Input: part model. Units: mm. Frame: model coordinates. A direction names the side the tool comes from. Coordinates: 2 decimals unless noted, no trailing zeros. Loops run counter-clockwise (first coordinate to the right, second up) from the corner with the lowest first, then second, coordinate; pieces in that order, holes last.
```python
from build123d import *

# Parameters (mm, degrees)
F0_R     = 5.3
F1_DEPTH = 3
F2_W     = 10.177304
F2_H     = 3
F3_DEPTH = 5
F4_R     = 1.5
F5_DEPTH = 5


with BuildPart() as f1:
    # F0 (on Top) → F1 (new body)
    with BuildSketch(Plane.XY):
        with BuildLine():
            Line((-12.261554, 0), (-20, 0))
            Line((-20, 0), (-20, -3))
            Line((-20, -3), (0, -3))
            Line((0, -3), (20, -3))
            Line((20, -3), (20, 0))
            Line((20, 0), (12.261554, 0))
            ThreePointArc((12.261554, 0), (8.853776, 1.888736), (7.485685, 5.536832))
            ThreePointArc((7.485685, 5.536832), (7.488618, 5.754393), (7.499947, 5.971679))
            ThreePointArc((7.499947, 5.971679), (0, 13.5), (-7.499947, 5.971679))
            ThreePointArc((-7.499947, 5.971679), (-7.488618, 5.754393), (-7.485685, 5.536832))
            ThreePointArc((-7.485685, 5.536832), (-8.853776, 1.888736), (-12.261554, 0))
        make_face()
        with Locations((0, 6)):
            Circle(F0_R, mode=Mode.SUBTRACT)
        with BuildLine():
            ThreePointArc((-7.499947, 5.971679), (-7.495969, 5.754152), (-7.485685, 5.536832))
            ThreePointArc((-7.485685, 5.536832), (-7.488618, 5.754393), (-7.499947, 5.971679))
        make_face()
        with BuildLine():
            ThreePointArc((7.485685, 5.536832), (7.495969, 5.754152), (7.499947, 5.971679))
            ThreePointArc((7.499947, 5.971679), (7.488618, 5.754393), (7.485685, 5.536832))
        make_face()
    extrude(amount=F1_DEPTH)

    # F2 (on face) → F3 (join)
    with BuildSketch(Plane(origin=(0, 0, 0), x_dir=(1, 0, 0), z_dir=(0, 0, -1))):
        with Locations((-14.911348, 1.5)):
            Rectangle(F2_W, F2_H)
        with Locations((14.911348, 1.5)):
            Rectangle(F2_W, F2_H)
    extrude(amount=F3_DEPTH)

    # F4 (on face) → F5 (cut)
    with BuildSketch(Plane(origin=(0, 0, 0), x_dir=(-1, 0, 0), z_dir=(0, 1, 0))):
        with Locations((-15, -2)):
            Circle(F4_R)
        with Locations((15, -2)):
            Circle(F4_R)
    extrude(amount=-F5_DEPTH, mode=Mode.SUBTRACT)


solid = f1.part
```
Item 1: Line query: L1, parallel to Z at x = 15, y = -1.75; L2, parallel to Y at x = 15.5, z = 0; L3, parallel to Y at x = 0, z = 1.55. Output: solid intervals per line, ascending.
Result:
L1: z = -5 to -3.5, -0.5 to 3
L2: y = -3 to 0
L3: y = -3 to 0.7, 11.3 to 13.5
Item 2: Section query D-D (y = 7.75). Output: boundary loops of the cut face in (x, z).
Result:
outline: (-7.29, 0) - (-5, 0) - (-5, 3) - (-7.29, 3) - close; (5, 0) - (7.29, 0) - (7.29, 3) - (5, 3) - close
Item 3: Reachability of faces 1 (the face through (-9.823, -1, -2)), 2 (the face through (-15, 0, 0)), 3 (the face through (16.5, -1.48, -1.93)) from +Z, -Z, +X, -X, +Y, -Y: full face, straight path, thin tool, end or side. Return the list, or none.
Result:
face 1: -Z, +Y, -Y
face 2: -Z, -X, +Y
face 3: +Y, -Y
Item 4: Contact query for flat-ended pins moving along their axis: P1, Ø2.5, axis at x = -13, z = -0.5, coming from the +Y side; P2, Ø1, axis at y = 1, z = 1, coming from the +X side; P3, Ø2, axis at x = -15, z = 1.5, coming from the +Y side; P4, Ø8, axis at x = 7.5, y = 1.5, coming from the -Z side. Output: stop coordinate, or through.
Result:
P1: stops at y = 0.08
P2: stops at x = 10.66
P3: stops at y = 0
P4: stops at z = -5
Item 5: Section query A-A (x = 15). Output: boundary loops of the cut face in (y, z), then the cut area to 3 significant figures.
Result:
outline: (-3, -5) - (0, -5) - (0, -3.5) - (-3, -3.5) - close; (-3, -0.5) - (0, -0.5) - (0, 3) - (-3, 3) - close
area: 15.0 mm2
Item 6: Mould query, pull axis Y, two halves, no side actions, for faces 4 (the face through (-13.5, -1.48, -1.93)), 5 (the face through (0, -3, 1)), 6 (the face through (-0.69, 11.255, 1.479)), 7 (the face through (15, 0, 0)). Classes: +Y half, -Y half, draft (parallel to the pull), parting line (faces both ways), or undercut.
Result:
face 4: draft
face 5: -Y half
face 6: undercut
face 7: +Y half
Item 7: Section query B-B (y = -1.75). Output: boundary loops of the cut face in (x, z).
Result:
outline: (-20, -5) - (-9.82, -5) - (-9.82, 0) - (9.82, 0) - (9.82, -5) - (20, -5) - (20, 3) - (-20, 3) - close; hole circle Ø3 at (-15, -2); hole circle Ø3 at (15, -2)
Item 8: Section query C-C (z = -1). Output: boundary loops of the cut face in (x, y), then the cut area to 3 significant figures.
Result:
outline: (-20, -3) - (-16.12, -3) - (-16.12, 0) - (-20, 0) - close; (-13.88, -3) - (-9.82, -3) - (-9.82, 0) - (-13.88, 0) - close; (9.82, -3) - (13.88, -3) - (13.88, 0) - (9.82, 0) - close; (16.12, -3) - (20, -3) - (20, 0) - (16.12, 0) - close
area: 47.6 mm2
